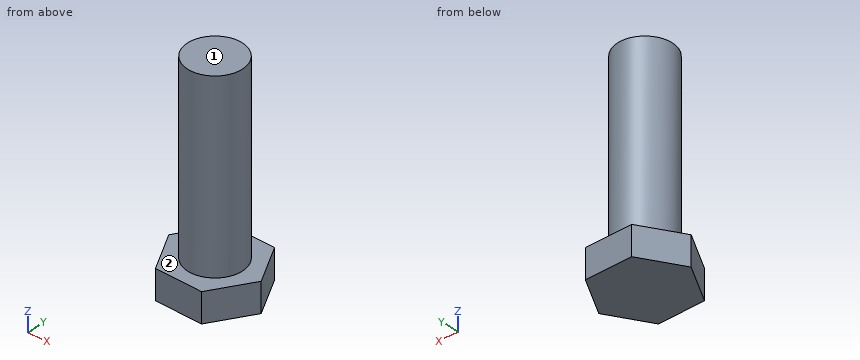
from build123d import *

# Parameters (mm, degrees)
EXTRUDE1_DEPTH    = 36.83
SKETCH2_OUTSIDE_W = 26.952
SKETCH2_OUTSIDE_H = 24.962
SKETCH2_OUTSIDE_R = 4.7625
EXTRUDE2_DEPTH    = 31.75


with BuildPart() as part:
    # Sketch1 → Extrude1 (new body)
    with BuildSketch(Plane.XY):
        Polygon((4.274924982, 6.994647743), (-3.920080145, 7.199517506), (-8.195005127, 0.204869763), (-4.274924982, -6.994647743), (3.920080145, -7.199517506), (8.195005127, -0.204869763), align=None)
    extrude(amount=EXTRUDE1_DEPTH)

    # Sketch2 outside → Extrude2 (cut)
    with BuildSketch(Plane.XY.offset(36.83)):
        Rectangle(SKETCH2_OUTSIDE_W, SKETCH2_OUTSIDE_H)
        Circle(SKETCH2_OUTSIDE_R, mode=Mode.SUBTRACT)
    extrude(amount=-EXTRUDE2_DEPTH, mode=Mode.SUBTRACT)


solid = part.part
Model file for the job. Use its own axes, mm. Face numbers are marked on the shaded views. A direction names the side the tool comes from. Round coordinates to 2 decimals unless told otherwise and drop trailing zeros. Loops run counter-clockwise (first coordinate to the right, second up) from the corner with the lowest first, then second, coordinate; pieces in that order, holes last. Notation, with made-up numbers: (17.25, 0) - (40.25, 0) arc R33 ccw to (40.25, 38) - close; hole circle Ø10 at (37, 32). An arc over 180 degrees is marked (long way). Write each question's results on one line, items separated by ' | '.
(1) Saw through at C-C, the plane z = 32.5. List the corners of the cut face in (x, y) (1 decimal), then the cut area to 3 significant figures.
Answer below:
outline: circle Ø9.5 at (0, 0) | area: 71.3 mm^2
(2) Saw through at D-D, the plane y = -6. List the corners of the cut face in (x, z), then the cut area to 3 significant figures.
Answer below:
outline: (-4.82, 0) - (4.65, 0) - (4.65, 5.08) - (-4.82, 5.08) - close | area: 48.1 mm^2
(3) Pin check, flat tips, straight feed: pin 1 (6 mm diameter, centred on x = -5, z = 29, fed in from -Y); pin 2 (6 mm diameter, centred on x = 3, z = 12.5, fed in from +Y); pin 3 (8 mm diameter, centred on x = -5.5, y = 4.5, fed in from -Z); pin 4 (3 mm diameter, centred on x = -6, z = 5, fed in from +Y). Stop position of each tip, or through.
Answer below:
pin 1: stops at y = -4.32 | pin 2: stops at y = 4.76 | pin 3: stops at z = 0 | pin 4: stops at y = 6.25
(4) Wall check: L1, parallel to Z at x = -6, y = 3.5; L2, parallel to X at y = -5.5, z = 3; L3, parallel to X at y = -2.75, z = 13.5. Give the ranges that are in metal, low to high.
Answer below:
L1: z = 0 to 5.08 | L2: x = -5.09 to 4.96 | L3: x = -3.89 to 3.89
(5) 3-axis set-ups, long thin cutter, end or side, ignore diameter. For the marked faces 1 and 2: which of +Z, -Z, +X, -X, +Y, -Y reach the whole face in a straight line?
Answer below:
face 1: +Z, +X, -X, +Y, -Y | face 2: +Z
(6) Saw through at A-A, the plane x = 1.25. List the corners of the cut face in (y, z).
Answer below:
outline: (-7.13, 0) - (7.07, 0) - (7.07, 5.08) - (4.6, 5.08) - (4.6, 36.83) - (-4.6, 36.83) - (-4.6, 5.08) - (-7.13, 5.08) - close
(7) Saw through at B-B, the plane y = 2.5. List the corners of the cut face in (x, z).
Answer below:
outline: (-6.79, 0) - (6.72, 0) - (6.72, 5.08) - (4.05, 5.08) - (4.05, 36.83) - (-4.05, 36.83) - (-4.05, 5.08) - (-6.79, 5.08) - close
